Build history of the part. All positions in model axes, mm. Face numbers are marked on the shaded views. A direction names the side the tool comes from. Coordinates: 2 decimals unless noted, no trailing zeros. Loops run counter-clockwise (first coordinate to the right, second up) from the corner with the lowest first, then second, coordinate; pieces in that order, holes last.
(1) Slice it at C-C (x = 38.5). Give the cut face in (y, z) (3 decimals), and give its area (3 significant figures).
(2) Wall check: L1, parallel to X at y = -7.25, z = 14.75; L2, parallel to X at y = 1, z = 18.25; L3, parallel to Y at x = 6.5, z = 11.25 (3 decimals). Give the ranges that are in metal, low to high.
(3) Slice it at A-A (z = 9). Give the number of separate pieces and of enclosed holes in the cut face, and give its area (3 significant figures).
(4) Slice it at B-B (y = 0). Give the cut face in (x, z).
(5) Flat gauge pins, fed straight in: P1, Ø3.5, axis at y = 10, z = 14.5, coming from the -X side; P2, Ø6, axis at x = 3.5, z = 9, coming from the -Y side (3 decimals); P3, Ø3, axis at x = 19, z = 14.5, coming from the +Y side (3 decimals); P4, Ø4, axis at x = -43.5, y = 0, coming from the +Z side. Where does each tip first touch, or does it go through?
(6) Two-plate mould, pull along X, no slides. Class the marked faces 5, 6 and 7: pulls with the +X half, pulls with the -X half, needs draft (parallel to the pull), parting line crosses it, or undercut.
(7) Tool access for the marked faces 1, 2, 3 and 4: list every direction of +Z, -Z, +X, -X, +Y, -Y with a clear straight run to the whole face (end or side of a thin tool).
from build123d import *

# Parameters (mm, degrees)
F0_R     = 2.25
F0_W     = 75
F0_H     = 16.75
F1_DEPTH = 16.75
F2_SIZE  = 1.5
F3_W     = 3
F3_H     = 11
F4_DEPTH = 3
F5_W     = 2
F5_H     = 10
F6_DEPTH = 2.5
F7_W     = 12.7
F7_H     = 6.4
F8_DEPTH = 25.9222812921
F9_SIZE  = 2.75


with BuildPart() as f1:
    # F0 (on Top) → F1 (new body)
    with BuildSketch(Plane.XY):
        Polygon((43.5, 6.4), (43.5, 11.575), (3.2, 11.575), (1.6, 14.3462812921), (-1.6, 14.3462812921), (-3.2, 11.575), (-43.5, 11.575), (-43.5, 6.4), (-49.0425625842, 3.2), (-49.0425625842, -3.2), (-43.5, -6.4), (-43.5, -11.575), (-23.2, -11.575), (-21.6, -14.3462812921), (-18.4, -14.3462812921), (-16.8, -11.575), (16.8, -11.575), (18.4, -14.3462812921), (21.6, -14.3462812921), (23.2, -11.575), (43.5, -11.575), (43.5, -6.4), (49.0425625842, -3.2), (49.0425625842, 3.2), align=None)
        with Locations((-43.5, 0)):
            Circle(F0_R, mode=Mode.SUBTRACT)
        Rectangle(F0_W, F0_H, mode=Mode.SUBTRACT)
        with Locations((43.5, 0)):
            Circle(F0_R, mode=Mode.SUBTRACT)
    extrude(amount=F1_DEPTH)

    # F2
    f2_edges = [f1.edges().sort_by_distance(p)[0] for p in [
        (-43.5, 11.575, 8.375),
        (43.5, 11.575, 8.375),
        (43.5, -11.575, 8.375),
        (-43.5, -11.575, 8.375),
    ]]
    chamfer(f2_edges, length=F2_SIZE)

    # F3 (on Top) → F4 (cut)
    with BuildSketch(Plane.XY):
        with Locations((-39, 0)):
            Rectangle(F3_W, F3_H)
        with Locations((39, 0)):
            Rectangle(F3_W, F3_H)
    extrude(amount=F4_DEPTH, mode=Mode.SUBTRACT)

    # F5 (on face) → F6 (join)
    with BuildSketch(Plane.XY.offset(16.75)):
        with Locations((-38.5, 0)):
            Rectangle(F5_W, F5_H)
        with Locations((38.5, 0)):
            Rectangle(F5_W, F5_H)
    extrude(amount=F6_DEPTH)

    # F7 (on face) → F8 (cut, through all)
    with BuildSketch(Plane.XZ.offset(11.575)):
        with Locations((0, 16.75)):
            Rectangle(F7_W, F7_H)
    extrude(amount=-F8_DEPTH, mode=Mode.SUBTRACT)

    # F9
    f9_edges = [f1.edges().sort_by_distance(p)[0] for p in [
        (0, 14.346281, 13.55),
    ]]
    chamfer(f9_edges, length=F9_SIZE)


solid = f1.part
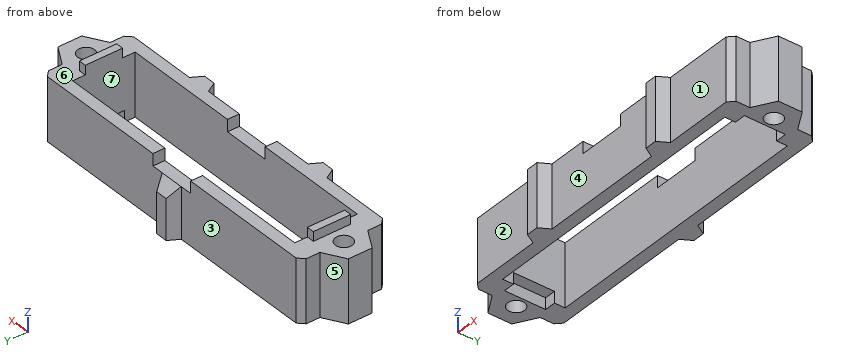
Response values:
1. outline: (-11.575, 0) - (-5.5, 0) - (-5.5, 3) - (5.5, 3) - (5.5, 0) - (11.575, 0) - (11.575, 16.75) - (5, 16.75) - (5, 19.25) - (-5, 19.25) - (-5, 16.75) - (-11.575, 16.75) - close
1. area: 380 mm2
2. L1: x = -43.5 to -37.5, 37.5 to 43.5
2. L2: x = -39.5 to -37.5, 37.5 to 39.5
2. L3: y = -11.575 to -8.375, 8.375 to 11.575
3. separate pieces: 1
3. enclosed holes: 3
3. area: 868 mm2
4. outline: (-49.04, 0) - (-45.75, 0) - (-45.75, 16.75) - (-49.04, 16.75) - close; (-41.25, 0) - (-40.5, 0) - (-40.5, 3) - (-37.5, 3) - (-37.5, 19.25) - (-39.5, 19.25) - (-39.5, 16.75) - (-41.25, 16.75) - close; (37.5, 3) - (40.5, 3) - (40.5, 0) - (41.25, 0) - (41.25, 16.75) - (39.5, 16.75) - (39.5, 19.25) - (37.5, 19.25) - close; (45.75, 0) - (49.04, 0) - (49.04, 16.75) - (45.75, 16.75) - close
5. P1: stops at x = -43.5
5. P2: stops at y = -11.575
5. P3: stops at y = 11.575
5. P4: passes through
6. face 5: pulls with the -X half
6. face 6: needs draft
6. face 7: undercut
7. face 1: +Z, -Z, +X, -Y
7. face 2: +Z, -Z, -X, -Y
7. face 3: +Z, -Z, -X, +Y
7. face 4: +Z, -Z, -Y
